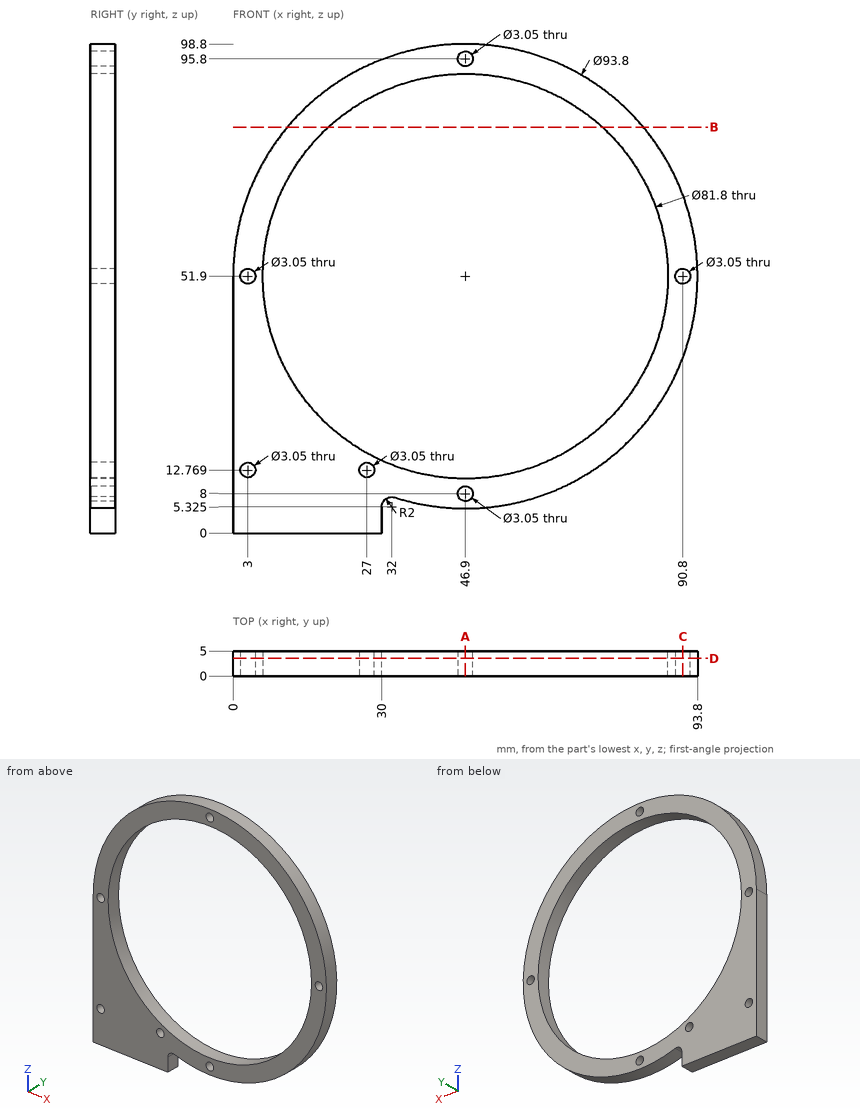
Input: dimensioned drawing with shaded views. Units: mm. Origin: part minimum x, y, z. Coordinates: 2 decimals unless noted, no trailing zeros. Loops run counter-clockwise (first coordinate to the right, second up) from the corner with the lowest first, then second, coordinate; pieces in that order, holes last. Notation, with made-up numbers: (89.25, 9.5) -> (99.25, 9.5) arc R12 ccw to (99.25, 29.5) -> close; hole circle Ø9 at (-2, 75.5). An arc over 180 degrees is marked (long way). One line per item, written item: value. Start each with the question number.
Q1. Section query D-D, the plane y = 3.55. Give the number of separate pieces and of enclosed holes in the cut face, and give its area (3 significant figures).
Q2. Line query: line 1 along X through (y, z) = (1.85, 51.9) (1 decimal); line 2 along X through (y, z) = (4.75, 14) (1 decimal); line 3 along Z through (x, y) = (46.9, 3.5) (1 decimal). Output: solid intervals per line, ascending.
Q3. Section query A-A, the plane x = 46.9. Return the cut outline in (y, z) (1 decimal), and give its area (3 significant figures).
Q4. Contact query for flat-ended pins moving along their axis: P1, Ø1.5, axis at y = 2.5, z = 1.5, coming from the +X side; P2, Ø3.5, axis at x = 3, z = 51.9, coming from the +Y side; P3, Ø2, axis at y = 4, z = 65, coming from the -X side; P4, Ø1.5, axis at x = 49.5, y = 1.5, coming from the -Z side. Output: stop coordinate, or through.
Q5. Section query C-C, the plane x = 90.8. Return the cut outline in (y, z) (1 decimal).
Q6. Section query B-B, the plane z = 82. Return the cut outline in (x, y).
Results:
1. separate pieces: 1
1. enclosed holes: 7
1. area: 2,220 mm^2
2. line 1: 0 to 1.5, 4.5 to 6, 87.8 to 89.3, 92.3 to 93.8
2. line 2: 0 to 2.1, 3.9 to 26.1, 27.9 to 31.5, 62.3 to 74.5
2. line 3: 5 to 6.5, 9.5 to 11, 92.8 to 94.3, 97.3 to 98.8
3. outline: (0, 5) -> (5, 5) -> (5, 6.5) -> (0, 6.5) -> close; (0, 9.5) -> (5, 9.5) -> (5, 11) -> (0, 11) -> close; (0, 92.8) -> (5, 92.8) -> (5, 94.3) -> (0, 94.3) -> close; (0, 97.3) -> (5, 97.3) -> (5, 98.8) -> (0, 98.8) -> close
3. area: 29.5 mm^2
4. P1: x = 30
4. P2: y = 5
4. P3: x = 1.59
4. P4: z = 5.04
5. outline: (0, 35.4) -> (5, 35.4) -> (5, 50.4) -> (0, 50.4) -> close; (0, 53.4) -> (5, 53.4) -> (5, 68.4) -> (0, 68.4) -> close
6. outline: (10.93, 0) -> (19.21, 0) -> (19.21, 5) -> (10.93, 5) -> close; (74.59, 0) -> (82.87, 0) -> (82.87, 5) -> (74.59, 5) -> close
